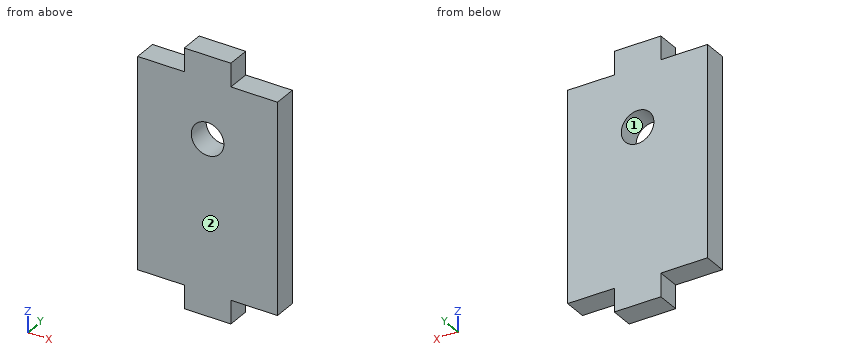
```python
from build123d import *

# Parameters (mm, degrees)
SKETCH1_R           = 3.5
SKETCH1_W           = 10
SKETCH1_H           = 5
BOSS_EXTRUDE1_DEPTH = 5


with BuildPart() as part:
    # Sketch1 → Boss-Extrude1 (new body)
    # profile 1 of 3: a face of its own
    with BuildSketch(Plane(origin=(0, 0, 0), x_dir=(1, 0, 0), z_dir=(0, 1, 0))):
        Polygon((15, -22.5), (15, 22.5), (5, 22.5), (-5, 22.5), (-15, 22.5), (-15, -22.5), (-5, -22.5), (5, -22.5), align=None)
        with Locations(Location((0, -9.9, 0), (0, 0, 270))):
            Circle(SKETCH1_R, mode=Mode.SUBTRACT)
    # profile 2 of 3: a face of its own
    with BuildSketch(Plane(origin=(0, 0, 0), x_dir=(1, 0, 0), z_dir=(0, 1, 0))):
        with Locations((0, -25)):
            Rectangle(SKETCH1_W, SKETCH1_H)
    # profile 3 of 3: a face of its own
    with BuildSketch(Plane(origin=(0, 0, 0), x_dir=(1, 0, 0), z_dir=(0, 1, 0))):
        with Locations((0, 25)):
            Rectangle(SKETCH1_W, SKETCH1_H)
    extrude(amount=BOSS_EXTRUDE1_DEPTH)


solid = part.part
```
Design review of the part built by this model. Coordinates are the model's own, in mm. Face numbers are marked on the shaded views. Coordinates: 2 decimals unless noted, no trailing zeros. Order: outer loops, then holes, each group sorted by start corner. A loop starts at its lowest first (then second) coordinate and runs counter-clockwise, first axis right, second up. Notation, with made-up numbers: (48.5, -19.5) - (60.5, -19.5) arc R27 ccw to (60.5, 4.5) - close; hole circle Ø4 at (86, 56). An arc over 180 degrees is marked (long way). Answer in a Markdown table with one row per item.
(1) Consider section D-D on x = 5.75. State the section outline as (y, z) points, plus the area to 3 significant figures.
Checked values:
| item | result |
|---|---|
| outline | (0, -22.5) - (5, -22.5) - (5, 22.5) - (0, 22.5) - close |
| area | 225 mm^2 |
(2) The part is to be moulded in two halves that separate along X. For the marked faces 1 and 2, say which applies: released by +X, released by -X, zero draft, split by the parting line, or undercut.
Checked values:
| item | result |
|---|---|
| face 1 | undercut |
| face 2 | zero draft |
(3) Wall thickness on line 1 along X through (y, z) = (3.5, 9.9); line 2 along Z through (x, y) = (13, 3.15); line 3 along Z through (x, y) = (-2, 4.75): over which ranges is each line inside the solid? List them lowest first. Write a range as from..to.
Checked values:
| item | result |
|---|---|
| line 1 | -15..-3.5, 3.5..15 |
| line 2 | -22.5..22.5 |
| line 3 | -27.5..7.03, 12.77..27.5 |
(4) Consider section A-A on y = 0.8. State the section outline as (x, z) points.
Checked values:
| item | result |
|---|---|
| outline | (-15, -22.5) - (-5, -22.5) - (-5, -27.5) - (5, -27.5) - (5, -22.5) - (15, -22.5) - (15, 22.5) - (5, 22.5) - (5, 27.5) - (-5, 27.5) - (-5, 22.5) - (-15, 22.5) - close; hole circle Ø7 at (0, 9.9) |
(5) Clearance check with flat-ended pins moving along their axes: pin 1 (1.5 mm diameter, centred on x = 11.5, y = 1.5, fed in from -Z); pin 2 (3 mm diameter, centred on x = 11.5, y = 1, fed in from +Z); pin 3 (9 mm diameter, centred on x = 0, z = 9.9, fed in from +Y); pin 4 (2.5 mm diameter, centred on y = 3.5, z = -25.5, fed in from +X). State where each tip first meets the part, or that it passes through.
Checked values:
| item | result |
|---|---|
| pin 1 | z = -22.5 |
| pin 2 | z = 22.5 |
| pin 3 | y = 5 |
| pin 4 | x = 5 |
(6) Consider section B-B on x = 0. State the section outline as (y, z) points.
Checked values:
| item | result |
|---|---|
| outline | (0, -27.5) - (5, -27.5) - (5, 6.4) - (0, 6.4) - close; (0, 13.4) - (5, 13.4) - (5, 27.5) - (0, 27.5) - close |
(7) Consider section C-C on z = 9.9. State the section outline as (x, y) points.
Checked values:
| item | result |
|---|---|
| outline | (-15, 0) - (-3.5, 0) - (-3.5, 5) - (-15, 5) - close; (3.5, 0) - (15, 0) - (15, 5) - (3.5, 5) - close |
